from build123d import *

# Parameters (mm, degrees)
BOSS_EXTRUDE1_DEPTH    = 6.35
F_10_CLEARANCE_HOLE1_D = 5.1054
CUT_EXTRUDE3_DEPTH     = 307.055384949
F_10_CLEARANCE_HOLE2_D = 5.1054
CUT_EXTRUDE4_DEPTH     = 307.055384949


with BuildPart() as part:
    # Sketch1 → Boss-Extrude1 (new body)
    with BuildSketch(Plane.XY):
        with BuildLine():
            Line((181.643586711, 23.126878769), (154.024056399, 149.054046391))
            ThreePointArc((154.024056399, 149.054046391), (157.752642202, 158.91005377), (168.275, 159.478578107))
            ThreePointArc((168.275, 159.478578107), (260.35, 0), (168.275, -159.478578107))
            ThreePointArc((168.275, -159.478578107), (157.752642202, -158.91005377), (154.024056399, -149.054046391))
            Line((154.024056399, -149.054046391), (181.643586711, -23.126878769))
            ThreePointArc((181.643586711, -23.126878769), (184.15, 0), (181.643586711, 23.126878769))
        make_face()
    extrude(amount=BOSS_EXTRUDE1_DEPTH)

    # #10 Clearance Hole1 (through all)
    with Locations(Plane(origin=(0, 0, 0), x_dir=(-1, 0, 0), z_dir=(0, 0, -1))):
        with Locations((-227.32143296, 87.25), (-250.7, 0), (-227.32143296, -87.25), (-163.45, 151.12143296), (-163.45, -151.12143296)):
            Hole(F_10_CLEARANCE_HOLE1_D / 2)

    # Sketch4 → Cut-Extrude3 (cut, through all)
    with BuildSketch(Plane(origin=(0, 0, 0), x_dir=(-1, 0, 0), z_dir=(0, 0, -1))):
        with BuildLine():
            Line((-228.389567551, -71.9105), (-180.764567551, -71.9105))
            ThreePointArc((-180.764567551, -71.9105), (-179.177067551, -70.323), (-177.589567551, -71.9105))
            Line((-177.589567551, -71.9105), (-177.589567551, -78.2605))
            ThreePointArc((-177.589567551, -78.2605), (-179.177067551, -79.848), (-180.764567551, -78.2605))
            Line((-180.764567551, -78.2605), (-228.389567551, -78.2605))
            ThreePointArc((-228.389567551, -78.2605), (-229.977067551, -79.848), (-231.564567551, -78.2605))
            Line((-231.564567551, -78.2605), (-231.564567551, -71.9105))
            ThreePointArc((-231.564567551, -71.9105), (-229.977067551, -70.323), (-228.389567551, -71.9105))
        make_face()
        with BuildLine():
            Line((-228.389567551, 78.2605), (-180.764567551, 78.2605))
            ThreePointArc((-180.764567551, 78.2605), (-179.177067551, 79.848), (-177.589567551, 78.2605))
            Line((-177.589567551, 78.2605), (-177.589567551, 71.9105))
            ThreePointArc((-177.589567551, 71.9105), (-179.177067551, 70.323), (-180.764567551, 71.9105))
            Line((-180.764567551, 71.9105), (-228.389567551, 71.9105))
            ThreePointArc((-228.389567551, 71.9105), (-229.977067551, 70.323), (-231.564567551, 71.9105))
            Line((-231.564567551, 71.9105), (-231.564567551, 78.2605))
            ThreePointArc((-231.564567551, 78.2605), (-229.977067551, 79.848), (-228.389567551, 78.2605))
        make_face()
    extrude(amount=-CUT_EXTRUDE3_DEPTH, mode=Mode.SUBTRACT)

    # #10 Clearance Hole2 (through all)
    with Locations(Plane(origin=(0, 0, 0), x_dir=(-1, 0, 0), z_dir=(0, 0, -1))):
        with Locations((-223.627067551, -50.8), (-185.527067551, 50.8), (-185.527067551, -50.8), (-223.627067551, 50.8)):
            Hole(F_10_CLEARANCE_HOLE2_D / 2)

    # Sketch7 → Cut-Extrude4 (cut, through all)
    with BuildSketch(Plane.XY.offset(6.35)):
        with BuildLine():
            Line((171.447975375, 128.892419043), (176.557773829, 105.595047978))
            ThreePointArc((176.557773829, 105.595047978), (180.372120431, 101.927081823), (185.220566537, 104.0474087))
            Line((185.220566537, 104.0474087), (193.878903814, 117.570865625))
            ThreePointArc((193.878903814, 117.570865625), (194.830328056, 121.796002086), (192.851503517, 125.648435037))
            ThreePointArc((192.851503517, 125.648435037), (187.306031839, 130.577762996), (181.552483119, 135.262547664))
            ThreePointArc((181.552483119, 135.262547664), (174.264118198, 135.62447632), (171.447975375, 128.892419043))
        make_face()
        with BuildLine():
            Line((194.823071175, 87.7855), (209.559327518, 87.7855))
            ThreePointArc((209.559327518, 87.7855), (213.147376547, 88.896377538), (215.480029332, 91.840333333))
            ThreePointArc((215.480029332, 91.840333333), (215.758641305, 92.502794413), (216.074279397, 93.148435108))
            ThreePointArc((216.074279397, 93.148435108), (216.785537654, 96.536247046), (215.614191178, 99.793716226))
            ThreePointArc((215.614191178, 99.793716226), (212.440037594, 104.085323924), (209.133824342, 108.276040036))
            ThreePointArc((209.133824342, 108.276040036), (203.848471686, 110.605496492), (198.862523013, 107.689740001))
            Line((198.862523013, 107.689740001), (190.81220141, 95.115942753))
            ThreePointArc((190.81220141, 95.115942753), (190.645079217, 90.262001434), (194.823071175, 87.7855))
        make_face()
        with BuildLine():
            Line((195.918284861, 36.653693121), (201.604222413, 21.491192982))
            ThreePointArc((201.604222413, 21.491192982), (204.577067551, 19.431009909), (207.54991269, 21.491192982))
            Line((207.54991269, 21.491192982), (213.235850242, 36.653693121))
            ThreePointArc((213.235850242, 36.653693121), (204.577067551, 49.148320597), (195.918284861, 36.653693121))
        make_face()
        with BuildLine():
            Line((221.69502961, 32.084292878), (214.666719976, 13.342133854))
            ThreePointArc((214.666719976, 13.342133854), (215.393182582, 7.49557278), (220.612410254, 4.7625))
            Line((220.612410254, 4.7625), (235.226963978, 4.7625))
            ThreePointArc((235.226963978, 4.7625), (238.125329178, 5.462546092), (240.384642652, 7.408333333))
            ThreePointArc((240.384642652, 7.408333333), (241.986845697, 9.239639717), (243.908896848, 10.731771428))
            ThreePointArc((243.908896848, 10.731771428), (246.218770536, 13.3100735), (246.833089321, 16.716797801))
            ThreePointArc((246.833089321, 16.716797801), (246.052937647, 23.346992794), (245.01525918, 29.941789658))
            ThreePointArc((245.01525918, 29.941789658), (234.172596645, 39.910658767), (221.69502961, 32.084292878))
        make_face()
        with BuildLine():
            Line((235.226963978, -4.7625), (220.612410254, -4.7625))
            ThreePointArc((220.612410254, -4.7625), (215.393182582, -7.49557278), (214.666719976, -13.342133854))
            Line((214.666719976, -13.342133854), (221.69502961, -32.084292878))
            ThreePointArc((221.69502961, -32.084292878), (234.172596645, -39.910658767), (245.01525918, -29.941789658))
            ThreePointArc((245.01525918, -29.941789658), (246.052937647, -23.346992794), (246.833089321, -16.716797801))
            ThreePointArc((246.833089321, -16.716797801), (246.218770536, -13.3100735), (243.908896848, -10.731771428))
            ThreePointArc((243.908896848, -10.731771428), (241.986845697, -9.239639717), (240.384642652, -7.408333333))
            ThreePointArc((240.384642652, -7.408333333), (238.125329178, -5.462546092), (235.226963978, -4.7625))
        make_face()
        with BuildLine():
            Line((213.235850242, -36.653693121), (207.54991269, -21.491192982))
            ThreePointArc((207.54991269, -21.491192982), (204.577067551, -19.431009909), (201.604222413, -21.491192982))
            Line((201.604222413, -21.491192982), (195.918284861, -36.653693121))
            ThreePointArc((195.918284861, -36.653693121), (204.577067551, -49.148320597), (213.235850242, -36.653693121))
        make_face()
        with BuildLine():
            Line((194.823071175, -87.7855), (209.559327518, -87.7855))
            ThreePointArc((209.559327518, -87.7855), (213.147376547, -88.896377538), (215.480029332, -91.840333333))
            ThreePointArc((215.480029332, -91.840333333), (215.758641305, -92.502794413), (216.074279397, -93.148435108))
            ThreePointArc((216.074279397, -93.148435108), (216.785537654, -96.536247046), (215.614191178, -99.793716226))
            ThreePointArc((215.614191178, -99.793716226), (212.440037594, -104.085323924), (209.133824342, -108.276040036))
            ThreePointArc((209.133824342, -108.276040036), (203.848471686, -110.605496492), (198.862523013, -107.689740001))
            Line((198.862523013, -107.689740001), (190.81220141, -95.115942753))
            ThreePointArc((190.81220141, -95.115942753), (190.645079217, -90.262001434), (194.823071175, -87.7855))
        make_face()
        with BuildLine():
            Line((185.220566537, -104.0474087), (193.878903814, -117.570865625))
            ThreePointArc((193.878903814, -117.570865625), (194.830328056, -121.796002086), (192.851503517, -125.648435037))
            ThreePointArc((192.851503517, -125.648435037), (187.306031839, -130.577762996), (181.552483119, -135.262547664))
            ThreePointArc((181.552483119, -135.262547664), (174.264118198, -135.62447632), (171.447975375, -128.892419043))
            Line((171.447975375, -128.892419043), (176.557773829, -105.595047978))
            ThreePointArc((176.557773829, -105.595047978), (180.372120431, -101.927081823), (185.220566537, -104.0474087))
        make_face()
    extrude(amount=-CUT_EXTRUDE4_DEPTH, mode=Mode.SUBTRACT)


solid = part.part
Part model, mm, in its own coordinate system. A direction names the side the tool comes from. Coordinates: 2 decimals unless noted, no trailing zeros. Loops run counter-clockwise (first coordinate to the right, second up) from the corner with the lowest first, then second, coordinate; pieces in that order, holes last. Notation, with made-up numbers: (10, 8) - (23, 8) arc R23 cw to (23, 30) - close; hole circle Ø11 at (12.5, 9). An arc over 180 degrees is marked (long way). Write each question's results on one line, items separated by ' | '. Start each with the question number.
Q1. Two-plate mould, pull along X, no slides. Class faces 1 (the cylindrical face through (157.88, -159, 3.13)), 2 (the flat face through (208, 2, 0)), 3 (the cylindrical face through (213.103, -88.866, 3.219)): +X half, -X half, draft (parallel to the pull), parting line (faces both ways), or undercut.
Q2. Probe line 1 along X through (y, z) = (-35, 0.5); line 2 along X through (y, z) = (71, 4); line 3 along Y through (x, z) = (235, 4.5). List the from-to ranges inside material, lowest first.
Q3. Slice it at A-A on z = 4. Give the number of separate pieces and of enclosed holes in the cut face, and give its area (3 significant figures).
Q4. Which spindle directions (+Z, -Z, +X, -X, +Y, -Y) get a long thin tool onto all of the face, cutting with end or side? Do faces 4 (the cylindrical face through (233.95, -39.93, 3.22)), 5 (the flat face through (208, 2, 6.35)). Say none if no direction does.
Q5. Drop flat-ended pins along their axis: pin 1 Ø1.5 at (x, z) = (230, 3.5) entering from +Y; pin 2 Ø3 at (y, z) = (75.5, 4) entering from -X; pin 3 Ø1.9 at (x, z) = (200, 4) entering from +Y. Give the stop position or say it passes through.
Q6. Slice it at B-B on y = -141. Give the cut face in (x, z).
Answer:
1) face 1: parting line | face 2: draft | face 3: undercut
2) line 1: x = 179.04 to 196.54, 212.62 to 223.27, 242.85 to 256.99 | line 2: x = 171.14 to 177.88, 180.48 to 228.68, 231.28 to 246.11 | line 3: y = -93.24 to -39.81, -4.76 to 4.76, 39.81 to 93.24
3) separate pieces: 1 | enclosed holes: 19 | area: 15,200 mm2
4) face 4: +Z, -Z | face 5: +Z, +X, -X, +Y, -Y
5) pin 1: stops at y = 102.41 | pin 2: stops at x = 169.83 | pin 3: stops at y = 137.18
6) outline: (155.79, 0) - (194.65, 0) - (194.65, 6.35) - (155.79, 6.35) - close
